from build123d import *

# Parameters (mm, degrees)
F0_W     = 25.4
F0_H     = 25.4
F1_DEPTH = 12.7
F3_W     = 25.4
F3_H     = 25.4
F5_R     = 5.08
F7_D     = 12.7
F7_DEPTH = 25.4
F7_TIP   = 3.8154649308
F9_D     = 12.7
F9_DEPTH = 25.4
F9_TIP   = 3.8154649308


with BuildPart() as f1:
    # F0 (on Top) → F1 (new body)
    with BuildSketch(Plane.XY):
        with BuildLine():
            Line((15.875, 0), (0, 0))
            ThreePointArc((0, 0), (-12.7, -12.7), (0, -25.4))
            Line((0, -25.4), (15.875, -25.4))
            Line((15.875, -25.4), (15.875, 0))
        make_face()
        with Locations((28.575, -12.7)):
            Rectangle(F0_W, F0_H)
        with BuildLine():
            Line((57.15, 0), (41.275, 0))
            Line((41.275, 0), (41.275, -25.4))
            Line((41.275, -25.4), (57.15, -25.4))
            ThreePointArc((57.15, -25.4), (69.85, -12.7), (57.15, 0))
        make_face()
    extrude(amount=F1_DEPTH)

    # F0 (on Top) → F4 section 0
    with BuildSketch(Plane.XY):
        with Locations((28.575, -12.7)):
            Rectangle(F0_W, F0_H)
    # F3 (on offset) → F4 section 1
    with BuildSketch(Plane.XY.offset(127)):
        with Locations((28.575, -12.7)):
            Rectangle(F3_W, F3_H)
    loft()

    # F5
    f5_edges = [f1.edges().sort_by_distance(p)[0] for p in [
        (41.275, -12.7, 12.7),
        (15.875, -12.7, 12.7),
        (28.575, 0, 127),
        (15.875, -12.7, 127),
        (28.575, -25.4, 127),
        (41.275, -12.7, 127),
    ]]
    fillet(f5_edges, radius=F5_R)

    # F7
    with Locations(Plane(origin=(0, 0, 0), x_dir=(1, 0, 0), z_dir=(0, 1, 0))):
        with Locations((28.575, -111.125)):
            Hole(F7_D / 2, depth=F7_DEPTH)
            with Locations((0, 0, -(F7_DEPTH + F7_TIP / 2))):  # 118° drill point
                Cone(0, F7_D / 2, F7_TIP, mode=Mode.SUBTRACT)

    # F9
    with Locations(Plane.XY.offset(12.7)):
        with Locations((-3.175, -12.7), (60.325, -12.7)):
            Hole(F9_D / 2, depth=F9_DEPTH)
            with Locations((0, 0, -(F9_DEPTH + F9_TIP / 2))):  # 118° drill point
                Cone(0, F9_D / 2, F9_TIP, mode=Mode.SUBTRACT)


solid = f1.part
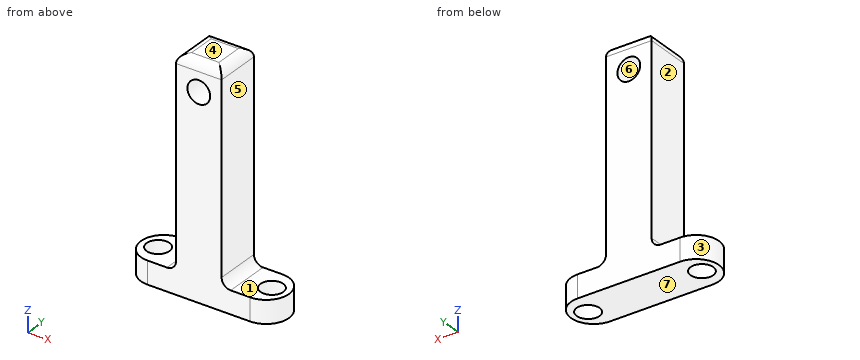
The listing builds one solid part. Answer for the finished solid, in the listing's coordinates (mm). Face numbers are marked on the shaded views. A direction names the side the tool comes from. Give positions to 0.01 mm unless a question says otherwise; leave off trailing zeros. Order: outer loops, then holes, each group sorted by start corner. A loop starts at its lowest first (then second) coordinate and runs counter-clockwise, first axis right, second up. Notation, with made-up numbers: (69, 79.5) - (100, 79.5) arc R13 ccw to (100, 97.5) - close; hole circle Ø10 at (51.5, -39). An arc over 180 degrees is marked (long way). One line per item, written item: value. Start each with the question number.
1) A cutting plane is placed at B-B on z = 106.5. Give the vertices of the cut face in (x, y) (3 decimals), then the cut area to 3 significant figures.
2) A cutting plane is placed at A-A on x = 28. Give the vertices of the cut face in (y, z), then the cut area to 3 significant figures.
3) A tool of negligible diameter and unlimited length cuts with its end or side. For the marked faces 1, 2 and 3, from which of +Z, -Z, +X, -X, +Y, -Y can it reach the whole face along a straight path? Write none if from no direction.
4) The mould has two halves that part along Z. Classify the marked faces 4, 5, 6 and 7: released by +Z, released by -Z, zero draft, split by the parting line, or undercut.
5) A cutting plane is placed at C-C on y = -17.75. Give the vertices of the cut face in (x, z) (3 decimals), then the cut area to 3 significant figures.
6) A cutting plane is placed at D-D on x = 7. Give the vertices of the cut face in (y, z), then the cut area to 3 significant figures.
7) Given pin 1 Ø7.5 at (y, z) = (-10.5, 95.5) entering from +X (3 decimals); pin 2 Ø12 at (x, y) = (-1, -22.5) entering from +Z; pin 3 Ø6 at (y, z) = (-11, 16.5) entering from -X, each flat-ended and moving along its own axis, determine where each tip first touches the part or whether it passes through.
8) Find the intervals of material crossed by L1, parallel to Z at x = 57.5, y = -22.75; L2, parallel to X at y = -4, z = 44 (3 decimals); L3, parallel to X at y = -7.25, z = 115.5 (3 decimals), in increasing order.
Answer sheet:
1. outline: (15.875, -25.4) - (24.224, -25.4) - (24.224, 0) - (15.875, 0) - close; (32.926, -25.4) - (41.275, -25.4) - (41.275, 0) - (32.926, 0) - close
1. area: 424 mm2
2. outline: (-25.4, 0) - (0, 0) - (0, 104.8) - (-25.4, 104.8) - close; (-25.4, 117.45) - (0, 117.45) - (0, 121.92) arc R5.08 ccw to (-5.08, 127) - (-20.32, 127) arc R5.08 ccw to (-25.4, 121.92) - close
2. area: 2,890 mm2
3. face 1: +Z, +X, +Y, -Y
3. face 2: +Z, -X, +Y, -Y
3. face 3: +Z, -Z, -X
4. face 4: released by +Z
4. face 5: zero draft
4. face 6: undercut
4. face 7: released by -Z
5. outline: (-11.653, 0) - (-7.025, 0) - (-7.025, 12.7) - (-11.653, 12.7) - close; (0.675, 0) - (56.475, 0) - (56.475, 12.7) - (46.355, 12.7) arc R5.08 cw to (41.275, 17.78) - (41.275, 121.92) arc R5.08 ccw to (36.195, 127) - (20.955, 127) arc R5.08 ccw to (15.875, 121.92) - (15.875, 17.78) arc R5.08 cw to (10.795, 12.7) - (0.675, 12.7) - close; (64.175, 0) - (68.803, 0) - (68.803, 12.7) - (64.175, 12.7) - close; hole circle Ø12.7 at (28.575, 111.125)
5. area: 3,600 mm2
6. outline: (-25.4, 0) - (0, 0) - (0, 12.7) - (-25.4, 12.7) - close
6. area: 323 mm2
7. pin 1: stops at x = 41.275
7. pin 2: stops at z = 12.7
7. pin 3: stops at x = 13.53
8. L1: z = 0 to 12.7
8. L2: x = 15.875 to 41.275
8. L3: x = 15.875 to 23.973, 33.177 to 41.275
